Build history of the part. All positions in model axes, mm. Face numbers are marked on the shaded views. A direction names the side the tool comes from. Give positions to 0.01 mm unless a question says otherwise; leave off trailing zeros. Loops run counter-clockwise (first coordinate to the right, second up) from the corner with the lowest first, then second, coordinate; pieces in that order, holes last. Notation, with made-up numbers: M -18.75,-23 L -8.75,-23 A30 ccw -8.75,6 Z; hole C 28,75 d5. An arc over 180 degrees is marked long. Answer as a JSON object with one key per item and string values. Group by question number.
1. Slice it at A-A (x = 42.5). List the corners of the cut face in (y, z), then the cut area to 3 significant figures.
2. 3-axis set-ups, long thin cutter, end or side, ignore diameter. For the marked faces 1, 2 and 3: which of +Z, -Z, +X, -X, +Y, -Y reach the whole face in a straight line?
3. Slice it at C-C (y = 4). List the corners of the cut face in (x, z), then the cut area to 3 significant figures.
4. Slice it at D-D (y = 26). List the corners of the cut face in (x, z), then the cut area to 3 significant figures.
5. Slice it at B-B (y = 19). List the corners of the cut face in (x, z).
6. Mould opens along Y. For the marked faces 4 and 5 say: released by +Y, released by -Y, zero draft, split by the parting line, or undercut.
7. Drop flat-ended pins along their axis: pin 1 Ø0.6 at (x, z) = (-2.5, 2.5) entering from -Y; pin 2 Ø3 at (x, y) = (-9, 15.5) entering from +Z; pin 3 Ø1.6 at (y, z) = (14, 3) entering from -X. Give the stop position or say it passes through.
8. Drill centre lines: line 1 along X through (y, z) = (13, 3.5); line 2 along Z through (x, y) = (-12, -4); line 3 along Y through (x, z) = (-5.5, 3). Where is each one in solid material? Low to high. Write a range as [from, to].
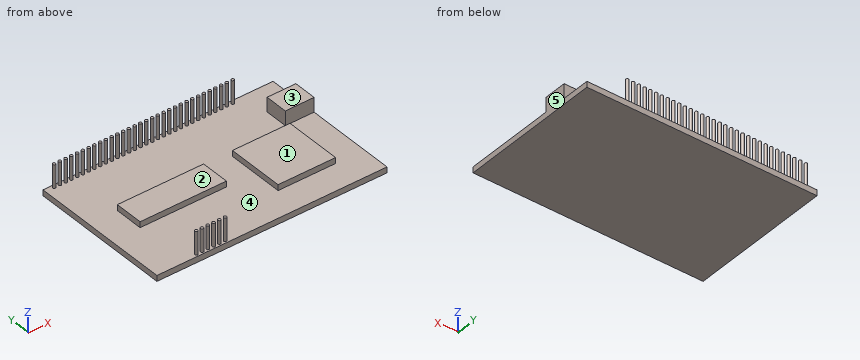
from build123d import *

# Parameters (mm, degrees)
SKETCH1_R           = 0.5
SKETCH1_W           = 30
SKETCH1_H           = 10
SKETCH1_W_2         = 20
SKETCH1_H_2         = 20
BOSS_EXTRUDE1_DEPTH = 2
SKETCH1_3_R         = 0.5
BOSS_EXTRUDE2_DEPTH = 10
SKETCH1_4_W         = 30
SKETCH1_4_H         = 10
SKETCH1_4_W_2       = 20
SKETCH1_4_H_2       = 20
BOSS_EXTRUDE3_DEPTH = 4
SKETCH1_5_W         = 10
SKETCH1_5_H         = 8
BOSS_EXTRUDE4_DEPTH = 7


with BuildPart() as part:
    # Sketch1 → Boss-Extrude1 (new body)
    with BuildSketch(Plane.XY):
        Polygon((51.15034045, 40.044862573), (-28.84965955, 40.044862573), (-28.84965955, -9.955137427), (51.15034045, -9.955137427), (51.15034045, 22.044862573), (41.15034045, 22.044862573), (41.15034045, 30.044862573), (51.15034045, 30.044862573), align=None)
        with Locations((-14.354824965, -8.955137427)):
            Circle(SKETCH1_R, mode=Mode.SUBTRACT)
        with Locations((-12.354824965, -8.955137427)):
            Circle(SKETCH1_R, mode=Mode.SUBTRACT)
        with Locations((-10.354824965, -8.955137427)):
            Circle(SKETCH1_R, mode=Mode.SUBTRACT)
        with Locations((-8.354824965, -8.955137427)):
            Circle(SKETCH1_R, mode=Mode.SUBTRACT)
        with Locations((-6.354824965, -8.955137427)):
            Circle(SKETCH1_R, mode=Mode.SUBTRACT)
        with Locations((-4.354824965, -8.955137427)):
            Circle(SKETCH1_R, mode=Mode.SUBTRACT)
        with Locations((-3.84965955, 15.044862573)):
            Rectangle(SKETCH1_W, SKETCH1_H, mode=Mode.SUBTRACT)
        with Locations((31.15034045, 10)):
            Rectangle(SKETCH1_W_2, SKETCH1_H_2, mode=Mode.SUBTRACT)
        with Locations((-25.767695538, 39.044862573)):
            Circle(SKETCH1_R, mode=Mode.SUBTRACT)
        with Locations((-23.767695538, 39.044862573)):
            Circle(SKETCH1_R, mode=Mode.SUBTRACT)
        with Locations((-21.767695538, 39.044862573)):
            Circle(SKETCH1_R, mode=Mode.SUBTRACT)
        with Locations((-19.767695538, 39.044862573)):
            Circle(SKETCH1_R, mode=Mode.SUBTRACT)
        with Locations((-17.767695538, 39.044862573)):
            Circle(SKETCH1_R, mode=Mode.SUBTRACT)
        with Locations((-15.767695538, 39.044862573)):
            Circle(SKETCH1_R, mode=Mode.SUBTRACT)
        with Locations((-13.767695538, 39.044862573)):
            Circle(SKETCH1_R, mode=Mode.SUBTRACT)
        with Locations((-11.767695538, 39.044862573)):
            Circle(SKETCH1_R, mode=Mode.SUBTRACT)
        with Locations((-9.767695538, 39.044862573)):
            Circle(SKETCH1_R, mode=Mode.SUBTRACT)
        with Locations((-7.767695538, 39.044862573)):
            Circle(SKETCH1_R, mode=Mode.SUBTRACT)
        with Locations((-5.767695538, 39.044862573)):
            Circle(SKETCH1_R, mode=Mode.SUBTRACT)
        with Locations((-3.767695538, 39.044862573)):
            Circle(SKETCH1_R, mode=Mode.SUBTRACT)
        with Locations((-1.767695538, 39.044862573)):
            Circle(SKETCH1_R, mode=Mode.SUBTRACT)
        with Locations((0.232304462, 39.044862573)):
            Circle(SKETCH1_R, mode=Mode.SUBTRACT)
        with Locations((2.232304462, 39.044862573)):
            Circle(SKETCH1_R, mode=Mode.SUBTRACT)
        with Locations((4.232304462, 39.044862573)):
            Circle(SKETCH1_R, mode=Mode.SUBTRACT)
        with Locations((6.264212791, 38.996436979)):
            Circle(SKETCH1_R, mode=Mode.SUBTRACT)
        with Locations((8.264212791, 38.996436979)):
            Circle(SKETCH1_R, mode=Mode.SUBTRACT)
        with Locations((10.264212791, 38.996436979)):
            Circle(SKETCH1_R, mode=Mode.SUBTRACT)
        with Locations((12.264212791, 38.996436979)):
            Circle(SKETCH1_R, mode=Mode.SUBTRACT)
        with Locations((14.264212791, 38.996436979)):
            Circle(SKETCH1_R, mode=Mode.SUBTRACT)
        with Locations((16.264212791, 38.996436979)):
            Circle(SKETCH1_R, mode=Mode.SUBTRACT)
        with Locations((18.264212791, 38.996436979)):
            Circle(SKETCH1_R, mode=Mode.SUBTRACT)
        with Locations((20.264212791, 38.996436979)):
            Circle(SKETCH1_R, mode=Mode.SUBTRACT)
        with Locations((22.264212791, 38.996436979)):
            Circle(SKETCH1_R, mode=Mode.SUBTRACT)
        with Locations((24.264212791, 38.996436979)):
            Circle(SKETCH1_R, mode=Mode.SUBTRACT)
        with Locations((26.264212791, 38.996436979)):
            Circle(SKETCH1_R, mode=Mode.SUBTRACT)
        with Locations((28.264212791, 38.996436979)):
            Circle(SKETCH1_R, mode=Mode.SUBTRACT)
        with Locations((30.264212791, 38.996436979)):
            Circle(SKETCH1_R, mode=Mode.SUBTRACT)
        with Locations((32.264212791, 38.996436979)):
            Circle(SKETCH1_R, mode=Mode.SUBTRACT)
        with Locations((34.264212791, 38.996436979)):
            Circle(SKETCH1_R, mode=Mode.SUBTRACT)
        with Locations((36.264212791, 38.996436979)):
            Circle(SKETCH1_R, mode=Mode.SUBTRACT)
    extrude(amount=BOSS_EXTRUDE1_DEPTH)

    # Sketch1<3> → Boss-Extrude2 (add)
    with BuildSketch(Plane.XY):
        with Locations((-25.767695538, 39.044862573)):
            Circle(SKETCH1_3_R)
        with Locations((-23.767695538, 39.044862573)):
            Circle(SKETCH1_3_R)
        with Locations((-19.767695538, 39.044862573)):
            Circle(SKETCH1_3_R)
        with Locations((-21.767695538, 39.044862573)):
            Circle(SKETCH1_3_R)
        with Locations((-17.767695538, 39.044862573)):
            Circle(SKETCH1_3_R)
        with Locations((-15.767695538, 39.044862573)):
            Circle(SKETCH1_3_R)
        with Locations((-13.767695538, 39.044862573)):
            Circle(SKETCH1_3_R)
        with Locations((-11.767695538, 39.044862573)):
            Circle(SKETCH1_3_R)
        with Locations((-14.354824965, -8.955137427)):
            Circle(SKETCH1_3_R)
        with Locations((-12.354824965, -8.955137427)):
            Circle(SKETCH1_3_R)
        with Locations((-10.354824965, -8.955137427)):
            Circle(SKETCH1_3_R)
        with Locations((-8.354824965, -8.955137427)):
            Circle(SKETCH1_3_R)
        with Locations((-6.354824965, -8.955137427)):
            Circle(SKETCH1_3_R)
        with Locations((-4.354824965, -8.955137427)):
            Circle(SKETCH1_3_R)
        with Locations((-9.767695538, 39.044862573)):
            Circle(SKETCH1_3_R)
        with Locations((-7.767695538, 39.044862573)):
            Circle(SKETCH1_3_R)
        with Locations((-5.767695538, 39.044862573)):
            Circle(SKETCH1_3_R)
        with Locations((-3.767695538, 39.044862573)):
            Circle(SKETCH1_3_R)
        with Locations((-1.767695538, 39.044862573)):
            Circle(SKETCH1_3_R)
        with Locations((2.232304462, 39.044862573)):
            Circle(SKETCH1_3_R)
        with Locations((0.232304462, 39.044862573)):
            Circle(SKETCH1_3_R)
        with Locations((4.232304462, 39.044862573)):
            Circle(SKETCH1_3_R)
        with Locations((6.264212791, 38.996436979)):
            Circle(SKETCH1_3_R)
        with Locations((8.264212791, 38.996436979)):
            Circle(SKETCH1_3_R)
        with Locations((10.264212791, 38.996436979)):
            Circle(SKETCH1_3_R)
        with Locations((12.264212791, 38.996436979)):
            Circle(SKETCH1_3_R)
        with Locations((14.264212791, 38.996436979)):
            Circle(SKETCH1_3_R)
        with Locations((16.264212791, 38.996436979)):
            Circle(SKETCH1_3_R)
        with Locations((18.264212791, 38.996436979)):
            Circle(SKETCH1_3_R)
        with Locations((20.264212791, 38.996436979)):
            Circle(SKETCH1_3_R)
        with Locations((22.264212791, 38.996436979)):
            Circle(SKETCH1_3_R)
        with Locations((24.264212791, 38.996436979)):
            Circle(SKETCH1_3_R)
        with Locations((26.264212791, 38.996436979)):
            Circle(SKETCH1_3_R)
        with Locations((28.264212791, 38.996436979)):
            Circle(SKETCH1_3_R)
        with Locations((30.264212791, 38.996436979)):
            Circle(SKETCH1_3_R)
        with Locations((32.264212791, 38.996436979)):
            Circle(SKETCH1_3_R)
        with Locations((36.264212791, 38.996436979)):
            Circle(SKETCH1_3_R)
        with Locations((34.264212791, 38.996436979)):
            Circle(SKETCH1_3_R)
    extrude(amount=BOSS_EXTRUDE2_DEPTH)

    # Sketch1<4> → Boss-Extrude3 (add)
    with BuildSketch(Plane.XY):
        with Locations((-3.84965955, 15.044862573)):
            Rectangle(SKETCH1_4_W, SKETCH1_4_H)
        with Locations((31.15034045, 10)):
            Rectangle(SKETCH1_4_W_2, SKETCH1_4_H_2)
    extrude(amount=BOSS_EXTRUDE3_DEPTH)

    # Sketch1<5> → Boss-Extrude4 (add)
    with BuildSketch(Plane.XY):
        with Locations((46.15034045, 26.044862573)):
            Rectangle(SKETCH1_5_W, SKETCH1_5_H)
    extrude(amount=BOSS_EXTRUDE4_DEPTH)


solid = part.part
Established:
{
 "1": {"outline": "M -9.96,0 L 40.04,0 L 40.04,2 L 30.04,2 L 30.04,7 L 22.04,7 L 22.04,2 L -9.96,2 Z", "area": "140 mm^2"},
 "2": {"face 1": "+Z, +X, -X, -Y", "face 2": "+Z, +X, -X", "face 3": "+Z, +X, -X, +Y, -Y"},
 "3": {"outline": "M -28.85,0 L 51.15,0 L 51.15,2 L 41.15,2 L 41.15,4 L 21.15,4 L 21.15,2 L -28.85,2 Z", "area": "200 mm^2"},
 "4": {"outline": "M -28.85,0 L 51.15,0 L 51.15,7 L 41.15,7 L 41.15,2 L -28.85,2 Z", "area": "210 mm^2"},
 "5": {"outline": "M -28.85,0 L 51.15,0 L 51.15,2 L 41.15,2 L 41.15,4 L 21.15,4 L 21.15,2 L 11.15,2 L 11.15,4 L -18.85,4 L -18.85,2 L -28.85,2 Z"},
 "6": {"face 4": "undercut", "face 5": "zero draft"},
 "7": {"pin 1": "stops at y = 10.04", "pin 2": "stops at z = 4", "pin 3": "stops at x = -18.85"},
 "8": {"line 1": "x = [-18.85, 11.15], [21.15, 41.15]", "line 2": "z = [0, 2]", "line 3": "y = [10.04, 20.04], [38.62, 39.47]"}
}
